Geometry check sheet. Reference: the model listing, model coordinates, mm. Coordinates: 2 decimals unless noted, no trailing zeros. Write each loop counter-clockwise with the first axis right and the second up, starting at its lowest first coordinate (ties: lowest second). Pieces come first, ordered by that corner, then holes. Notation, with made-up numbers: (16, 8.25) -> (43, 8.25) arc R30 cw to (43, 40.25) -> close; hole circle Ø4 at (54, 88.5). An arc over 180 degrees is marked (long way). Answer in a Markdown table with one row per item. Add a question column.
Q1. Gauge pin test, flat ends, axial feed: P1, Ø1.5, axis at x = 183, y = 224.5, coming from the +Z side; P2, Ø4, axis at x = 192, y = 109.5, coming from the +Z side; P3, Ø3, axis at x = 206.5, z = 8.5, coming from the -Y side; P4, Ø1.5, axis at x = 157.5, z = 4.5, coming from the -Y side. Record the tip position at first contact, or that the pin passes through.
Q2. Thickness scan on line 1 (X direction, y = 230, z = 3); line 2 (Y direction, x = 0, z = 5.5); line 3 (X direction, y = 156, z = 3.25). Record the ranges inside material, lowest first.
Q3. Section check B-B, the plane x = 0. Record the boundary of the cut face in (y, z).
Q4. Section check C-C, the plane x = 99.5. Record the boundary of the cut face in (y, z), and give its area (3 significant figures).
Q5. Section check A-A, the plane y = 53.5. Record the boundary of the cut face in (x, z).
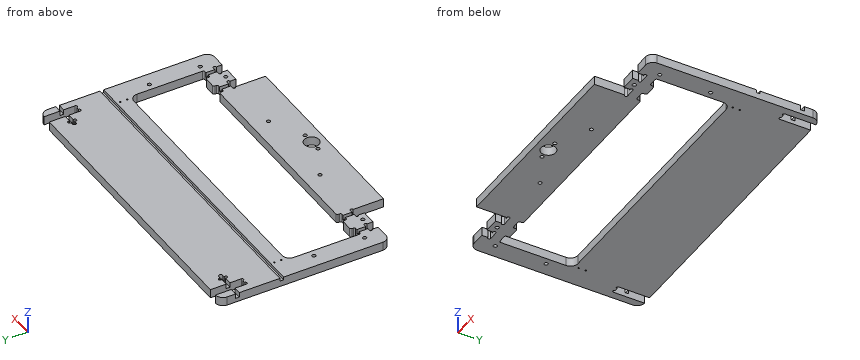
```python
from build123d import *

# Parameters (mm, degrees)
SKETCH1_W                = 275
SKETCH1_H                = 33
BOSS_EXTRUDE1_DEPTH      = 12
CUT_EXTRUDE1_REACH       = 141.005
SKETCH2_R                = 10
SKETCH2_R_2              = 2.5
SKETCH3_W                = 366
SKETCH3_H                = 95
BOSS_EXTRUDE2_DEPTH      = 12
CUT_EXTRUDE3_REACH       = 326.808
SKETCH5_W                = 14
SKETCH5_H                = 6
FILLET1_R                = 2
FILLET1_OF_MIRROR2_R     = 2
CUT_EXTRUDE6_REACH       = 326.808
SKETCH8_W                = 12
SKETCH8_H                = 42
F_5_0_5_DIAMETER_HOLE2_D = 5
CUT_EXTRUDE9_DEPTH       = 8
CUT_EXTRUDE10_DEPTH      = 6.5
F_5_0_5_DIAMETER_HOLE1_D = 5
F_2_0_2_DIAMETER_HOLE1_D = 2
SKETCH21_W               = 446.80085783
SKETCH21_H               = 5
CUT_EXTRUDE7_DEPTH       = 4
FILLET2_R                = 10
SKETCH25_W               = 5
SKETCH25_H               = 24
CUT_EXTRUDE11_DEPTH      = 6.5
CUT_EXTRUDE12_REACH      = 326.808
CUT_EXTRUDE13_REACH      = 326.808
SKETCH27_R               = 2


with BuildPart() as part:
    # Sketch1 → Boss-Extrude1 (new body)
    with BuildSketch(Plane.XY):
        Rectangle(SKETCH1_W, SKETCH1_H)
    extrude(amount=BOSS_EXTRUDE1_DEPTH)

    # Sketch2 → Cut-Extrude1 (cut, up to next)
    with BuildSketch(Plane.XY.offset(12), mode=Mode.PRIVATE) as cut_extrude1_sk1:
        with Locations((0, 1)):
            Circle(SKETCH2_R)
    cut_extrude1_tool1 = extrude(cut_extrude1_sk1.sketch, amount=-CUT_EXTRUDE1_REACH, mode=Mode.PRIVATE) & part.part
    # Sketch2 → Cut-Extrude1 (cut, up to next)
    with BuildSketch(Plane.XY.offset(12), mode=Mode.PRIVATE) as cut_extrude1_sk2:
        with Locations((-15, 1)):
            Circle(SKETCH2_R_2)
    cut_extrude1_tool2 = extrude(cut_extrude1_sk2.sketch, amount=-CUT_EXTRUDE1_REACH, mode=Mode.PRIVATE) & part.part
    # Sketch2 → Cut-Extrude1 (cut, up to next)
    with BuildSketch(Plane.XY.offset(12), mode=Mode.PRIVATE) as cut_extrude1_sk3:
        with Locations((15, 1)):
            Circle(SKETCH2_R_2)
    cut_extrude1_tool3 = extrude(cut_extrude1_sk3.sketch, amount=-CUT_EXTRUDE1_REACH, mode=Mode.PRIVATE) & part.part
    add(cut_extrude1_tool1.solids().sort_by_distance((0, 1, 12))[0], mode=Mode.SUBTRACT)
    add(cut_extrude1_tool2.solids().sort_by_distance((-15, 1, 12))[0], mode=Mode.SUBTRACT)
    add(cut_extrude1_tool3.solids().sort_by_distance((15, 1, 12))[0], mode=Mode.SUBTRACT)

    # Sketch3 → Boss-Extrude2 (add)
    with BuildSketch(Plane.XY.offset(12)):
        Polygon((-210, 16.5), (210, 16.5), (210, 46.5), (210, 247.5), (-210, 247.5), (-210, 46.5), align=None)
        with Locations((0, 94)):
            Rectangle(SKETCH3_W, SKETCH3_H, mode=Mode.SUBTRACT)
    extrude(amount=-BOSS_EXTRUDE2_DEPTH)

    # Sketch5 → Cut-Extrude3 (cut, up to next)
    with BuildSketch(Plane.XY.offset(12), mode=Mode.PRIVATE) as cut_extrude3_sk1:
        with Locations((-176, 43.5)):
            Rectangle(SKETCH5_W, SKETCH5_H)
    cut_extrude3_tool1 = extrude(cut_extrude3_sk1.sketch, amount=-CUT_EXTRUDE3_REACH, mode=Mode.PRIVATE) & part.part
    # Sketch5 → Cut-Extrude3 (cut, up to next)
    with BuildSketch(Plane.XY.offset(12), mode=Mode.PRIVATE) as cut_extrude3_sk2:
        with Locations((-144, 43.5)):
            Rectangle(SKETCH5_W, SKETCH5_H)
    cut_extrude3_tool2 = extrude(cut_extrude3_sk2.sketch, amount=-CUT_EXTRUDE3_REACH, mode=Mode.PRIVATE) & part.part
    cut_extrude3_1 = cut_extrude3_tool1.solids().sort_by_distance((-176, 43.5, 12))[0]
    add(cut_extrude3_1, mode=Mode.SUBTRACT)
    cut_extrude3_2 = cut_extrude3_tool2.solids().sort_by_distance((-144, 43.5, 12))[0]
    add(cut_extrude3_2, mode=Mode.SUBTRACT)
    cut_extrude3 = cut_extrude3_1 + cut_extrude3_2  # Cut-Extrude3 as one shape, for the pattern or mirror that repeats it

    # Fillet1
    fillet1_edges = [part.edges().sort_by_distance(p)[0] for p in [
        (-169, 46.5, 6),
        (-169, 40.5, 6),
        (-183, 40.5, 6),
        (-151, 46.5, 6),
        (-137, 46.5, 6),
        (-137, 40.5, 6),
        (-151, 40.5, 6),
    ]]
    fillet(fillet1_edges, radius=FILLET1_R)

    # Mirror2: Cut-Extrude3 across plane
    add(cut_extrude3.mirror(Plane(origin=(0, 0, 0), x_dir=(0, 0, 1), z_dir=(1, 0, 0))), mode=Mode.SUBTRACT)

    # Fillet1 of Mirror2
    fillet1_of_mirror2_edges = [part.edges().sort_by_distance(p)[0] for p in [
        (169, 46.5, 6),
        (169, 40.5, 6),
        (183, 40.5, 6),
        (151, 46.5, 6),
        (137, 46.5, 6),
        (137, 40.5, 6),
        (151, 40.5, 6),
    ]]
    fillet(fillet1_of_mirror2_edges, radius=FILLET1_OF_MIRROR2_R)

    # Sketch8 → Cut-Extrude6 (cut, up to next)
    with BuildSketch(Plane.XY.offset(12), mode=Mode.PRIVATE) as cut_extrude6_sk1:
        with Locations((-194, 226.5)):
            Rectangle(SKETCH8_W, SKETCH8_H)
    cut_extrude6_tool1 = extrude(cut_extrude6_sk1.sketch, amount=-CUT_EXTRUDE6_REACH, mode=Mode.PRIVATE) & part.part
    # Sketch8 → Cut-Extrude6 (cut, up to next)
    with BuildSketch(Plane.XY.offset(12), mode=Mode.PRIVATE) as cut_extrude6_sk2:
        with Locations((194, 226.5)):
            Rectangle(SKETCH8_W, SKETCH8_H)
    cut_extrude6_tool2 = extrude(cut_extrude6_sk2.sketch, amount=-CUT_EXTRUDE6_REACH, mode=Mode.PRIVATE) & part.part
    add(cut_extrude6_tool1.solids().sort_by_distance((-194, 226.5, 12))[0], mode=Mode.SUBTRACT)
    add(cut_extrude6_tool2.solids().sort_by_distance((194, 226.5, 12))[0], mode=Mode.SUBTRACT)

    # Ø5.0 (5) Diameter Hole2 (through all)
    with Locations(Plane(origin=(0, 0, 0), x_dir=(-1, 0, 0), z_dir=(0, 0, -1))):
        with Locations((192, 109.5), (192, 40.5)):
            f_5_0_5_diameter_hole2 = Hole(F_5_0_5_DIAMETER_HOLE2_D / 2)

    # Mirror3: Ø5.0 (5) Diameter Hole2 across plane
    add(f_5_0_5_diameter_hole2.mirror(Plane(origin=(0, 0, 0), x_dir=(0, 0, 1), z_dir=(1, 0, 0))), mode=Mode.SUBTRACT)

    # Sketch23 → Cut-Extrude9 (cut)
    with BuildSketch(Plane.XY.offset(12)):
        with BuildLine():
            Line((-178, 219.5), (-178, 227.5))
            ThreePointArc((-178, 227.5), (-176, 229.5), (-174, 227.5))
            Line((-174, 227.5), (-174, 219.5))
            ThreePointArc((-174, 219.5), (-176, 217.5), (-178, 219.5))
        make_face()
    cut_extrude9 = extrude(amount=-CUT_EXTRUDE9_DEPTH, mode=Mode.SUBTRACT)

    # Sketch24 → Cut-Extrude10 (cut)
    with BuildSketch(Plane.XY.offset(12)):
        with BuildLine():
            Line((-222.733424796, 226), (-171, 226))
            ThreePointArc((-171, 226), (-168.5, 223.5), (-171, 221))
            Line((-171, 221), (-222.733424796, 221))
            ThreePointArc((-222.733424796, 221), (-225.233424796, 223.5), (-222.733424796, 226))
        make_face()
    cut_extrude10 = extrude(amount=-CUT_EXTRUDE10_DEPTH, mode=Mode.SUBTRACT)

    # Ø5.0 (5) Diameter Hole1 (through all)
    with Locations(Plane(origin=(0, 0, 0), x_dir=(-1, 0, 0), z_dir=(0, 0, -1))):
        with Locations((-60, 24.5), (60, 24.5), (160, 24.5), (-160, 24.5)):
            Hole(F_5_0_5_DIAMETER_HOLE1_D / 2)

    # Ø2.0 (2) Diameter Hole1 (through all)
    with Locations(Plane.XY.offset(12)):
        with Locations((-180, 156), (-180, 146.5)):
            f_2_0_2_diameter_hole1 = Hole(F_2_0_2_DIAMETER_HOLE1_D / 2)

    # Mirror4: Cut-Extrude9, Cut-Extrude10, Ø2.0 (2) Diameter Hole1 across plane
    add(cut_extrude9.mirror(Plane(origin=(0, 0, 0), x_dir=(0, 0, 1), z_dir=(1, 0, 0))), mode=Mode.SUBTRACT)
    add(cut_extrude10.mirror(Plane(origin=(0, 0, 0), x_dir=(0, 0, 1), z_dir=(1, 0, 0))), mode=Mode.SUBTRACT)
    add(f_2_0_2_diameter_hole1.mirror(Plane(origin=(0, 0, 0), x_dir=(0, 0, 1), z_dir=(1, 0, 0))), mode=Mode.SUBTRACT)

    # Sketch21 → Cut-Extrude7 (cut)
    with BuildSketch(Plane.XY.offset(12)):
        with Locations((9.659590627, 163.5)):
            Rectangle(SKETCH21_W, SKETCH21_H)
    extrude(amount=-CUT_EXTRUDE7_DEPTH, mode=Mode.SUBTRACT)

    # Fillet2
    fillet2_edges = [part.edges().sort_by_distance(p)[0] for p in [
        (210, 247.5, 6),
        (210, 16.5, 6),
        (-210, 16.5, 6),
        (-210, 247.5, 6),
        (183, 141.5, 6),
        (-183, 141.5, 6),
    ]]
    fillet(fillet2_edges, radius=FILLET2_R - 0.0001)  # a hair under: the kernel refuses the full size

    # Sketch25 → Cut-Extrude11 (cut)
    with BuildSketch(Plane.XY.offset(12)):
        with Locations((-176, 40.5)):
            Rectangle(SKETCH25_W, SKETCH25_H)
        with Locations((-144, 40.5)):
            Rectangle(SKETCH25_W, SKETCH25_H)
    cut_extrude11 = extrude(amount=-CUT_EXTRUDE11_DEPTH, mode=Mode.SUBTRACT)

    # Sketch26 → Cut-Extrude12 (cut, up to next)
    with BuildSketch(Plane.XY.offset(12), mode=Mode.PRIVATE) as cut_extrude12_sk1:
        with BuildLine():
            Line((-182, 16.5), (-170, 16.5))
            Line((-170, 16.5), (-170, 24.5))
            ThreePointArc((-170, 24.5), (-168, 26.5), (-170, 28.5))
            Line((-170, 28.5), (-182, 28.5))
            ThreePointArc((-182, 28.5), (-184, 26.5), (-182, 24.5))
            Line((-182, 24.5), (-182, 16.5))
        make_face()
    cut_extrude12_tool1 = extrude(cut_extrude12_sk1.sketch, amount=-CUT_EXTRUDE12_REACH, mode=Mode.PRIVATE) & part.part
    # Sketch26 → Cut-Extrude12 (cut, up to next)
    with BuildSketch(Plane.XY.offset(12), mode=Mode.PRIVATE) as cut_extrude12_sk2:
        with BuildLine():
            Line((-150, 16.5), (-137.5, 16.5))
            Line((-137.5, 16.5), (-137.5, 24.5))
            ThreePointArc((-137.5, 24.5), (-135.5, 26.5), (-137.5, 28.5))
            Line((-137.5, 28.5), (-150, 28.5))
            ThreePointArc((-150, 28.5), (-152, 26.5), (-150, 24.5))
            Line((-150, 24.5), (-150, 16.5))
        make_face()
    cut_extrude12_tool2 = extrude(cut_extrude12_sk2.sketch, amount=-CUT_EXTRUDE12_REACH, mode=Mode.PRIVATE) & part.part
    cut_extrude12_1 = cut_extrude12_tool1.solids().sort_by_distance((-176, 22.821049, 12))[0]
    add(cut_extrude12_1, mode=Mode.SUBTRACT)
    cut_extrude12_2 = cut_extrude12_tool2.solids().sort_by_distance((-143.75, 22.8092, 12))[0]
    add(cut_extrude12_2, mode=Mode.SUBTRACT)
    cut_extrude12 = cut_extrude12_1 + cut_extrude12_2  # Cut-Extrude12 as one shape, for the pattern or mirror that repeats it

    # Mirror5: Cut-Extrude11, Cut-Extrude12 across plane
    add(cut_extrude11.mirror(Plane(origin=(0, 0, 0), x_dir=(0, 0, 1), z_dir=(1, 0, 0))), mode=Mode.SUBTRACT)
    add(cut_extrude12.mirror(Plane(origin=(0, 0, 0), x_dir=(0, 0, 1), z_dir=(1, 0, 0))), mode=Mode.SUBTRACT)

    # Sketch27 → Cut-Extrude13 (cut, up to next)
    with BuildSketch(Plane.XY.offset(12), mode=Mode.PRIVATE) as cut_extrude13_sk1:
        with Locations((-198, 205.5)):
            Circle(SKETCH27_R)
    cut_extrude13_tool1 = extrude(cut_extrude13_sk1.sketch, amount=-CUT_EXTRUDE13_REACH, mode=Mode.PRIVATE) & part.part
    # Sketch27 → Cut-Extrude13 (cut, up to next)
    with BuildSketch(Plane.XY.offset(12), mode=Mode.PRIVATE) as cut_extrude13_sk2:
        with Locations((-190, 205.5)):
            Circle(SKETCH27_R)
    cut_extrude13_tool2 = extrude(cut_extrude13_sk2.sketch, amount=-CUT_EXTRUDE13_REACH, mode=Mode.PRIVATE) & part.part
    # Sketch27 → Cut-Extrude13 (cut, up to next)
    with BuildSketch(Plane.XY.offset(12), mode=Mode.PRIVATE) as cut_extrude13_sk3:
        with Locations((190, 205.5)):
            Circle(SKETCH27_R)
    cut_extrude13_tool3 = extrude(cut_extrude13_sk3.sketch, amount=-CUT_EXTRUDE13_REACH, mode=Mode.PRIVATE) & part.part
    # Sketch27 → Cut-Extrude13 (cut, up to next)
    with BuildSketch(Plane.XY.offset(12), mode=Mode.PRIVATE) as cut_extrude13_sk4:
        with Locations((198, 205.5)):
            Circle(SKETCH27_R)
    cut_extrude13_tool4 = extrude(cut_extrude13_sk4.sketch, amount=-CUT_EXTRUDE13_REACH, mode=Mode.PRIVATE) & part.part
    add(cut_extrude13_tool1.solids().sort_by_distance((-198, 205.5, 12))[0], mode=Mode.SUBTRACT)
    add(cut_extrude13_tool2.solids().sort_by_distance((-190, 205.5, 12))[0], mode=Mode.SUBTRACT)
    add(cut_extrude13_tool3.solids().sort_by_distance((190, 205.5, 12))[0], mode=Mode.SUBTRACT)
    add(cut_extrude13_tool4.solids().sort_by_distance((198, 205.5, 12))[0], mode=Mode.SUBTRACT)


solid = part.part
```
Calculated:
| question | item | result |
|---|---|---|
| 1 | P1 | stops at z = 5.5 |
| 1 | P2 | passes through |
| 1 | P3 | stops at y = 17.84 |
| 1 | P4 | stops at y = 16.5 |
| 2 | line 1 | x = -210 to -200, -188 to 188, 200 to 210 |
| 2 | line 2 | y = -16.5 to -9, 11 to 46.5, 141.5 to 247.5 |
| 2 | line 3 | x = -210 to -181, -179 to 179, 181 to 210 |
| 3 | outline | (-16.5, 0) -> (-9, 0) -> (-9, 12) -> (-16.5, 12) -> close; (11, 0) -> (46.5, 0) -> (46.5, 12) -> (11, 12) -> close; (141.5, 0) -> (247.5, 0) -> (247.5, 12) -> (166, 12) -> (166, 8) -> (161, 8) -> (161, 12) -> (141.5, 12) -> close |
| 4 | outline | (-16.5, 0) -> (46.5, 0) -> (46.5, 12) -> (-16.5, 12) -> close; (141.5, 0) -> (247.5, 0) -> (247.5, 12) -> (166, 12) -> (166, 8) -> (161, 8) -> (161, 12) -> (141.5, 12) -> close |
| 4 | area | 2,010 mm² |
| 5 | outline | (-210, 0) -> (-183, 0) -> (-183, 12) -> (-210, 12) -> close; (183, 0) -> (210, 0) -> (210, 12) -> (183, 12) -> close |
